```python
from build123d import *

# Parameters (mm, degrees)
F0_W     = 76.2
F0_H     = 50.8
F0_R     = 12.7
F1_DEPTH = 12.7
F2_W     = 6.35
F2_H     = 50.8
F3_DEPTH = 2.54
F5_DEPTH = 50.8
F6_R     = 3.175
F7_DEPTH = 12.7


with BuildPart() as f1:
    # F0 (on Top) → F1 (new body)
    with BuildSketch(Plane.XY):
        Rectangle(F0_W, F0_H)
        Circle(F0_R, mode=Mode.SUBTRACT)
    extrude(amount=F1_DEPTH)

    # F2 (on face) → F3 (cut)
    with BuildSketch(Plane.XY.offset(12.7)):
        with BuildLine():
            ThreePointArc((6.35, 10.9985226281), (0, 12.7), (-6.35, 10.9985226281))
            Line((-6.35, 10.9985226281), (-6.35, -10.9985226281))
            ThreePointArc((-6.35, -10.9985226281), (0, -12.7), (6.35, -10.9985226281))
            Line((6.35, -10.9985226281), (6.35, 10.9985226281))
        make_face()
        with Locations((-32.385, 0)):
            Rectangle(F2_W, F2_H)
        with BuildLine():
            Line((-6.35, -10.9985226281), (-6.35, -25.4))
            Line((-6.35, -25.4), (6.35, -25.4))
            Line((6.35, -25.4), (6.35, -10.9985226281))
            ThreePointArc((6.35, -10.9985226281), (0, -12.7), (-6.35, -10.9985226281))
        make_face()
        with BuildLine():
            Line((6.35, 25.4), (-6.35, 25.4))
            Line((-6.35, 25.4), (-6.35, 10.9985226281))
            ThreePointArc((-6.35, 10.9985226281), (0, 12.7), (6.35, 10.9985226281))
            Line((6.35, 10.9985226281), (6.35, 25.4))
        make_face()
    extrude(amount=-F3_DEPTH, mode=Mode.SUBTRACT)

    # F4 (on face) → F5 (cut, through all)
    with BuildSketch(Plane.XZ.offset(25.4)):
        Polygon((31.75, 12.7), (19.05, 12.7), (16.1170606325, 7.62), (34.6829393675, 7.62), align=None)
    extrude(amount=-F5_DEPTH, mode=Mode.SUBTRACT)

    # F6 (on face) → F7 (join)
    with BuildSketch(Plane.YZ.offset(38.1)):
        with Locations((0, 6.35)):
            Circle(F6_R)
    extrude(amount=F7_DEPTH)


solid = f1.part
```
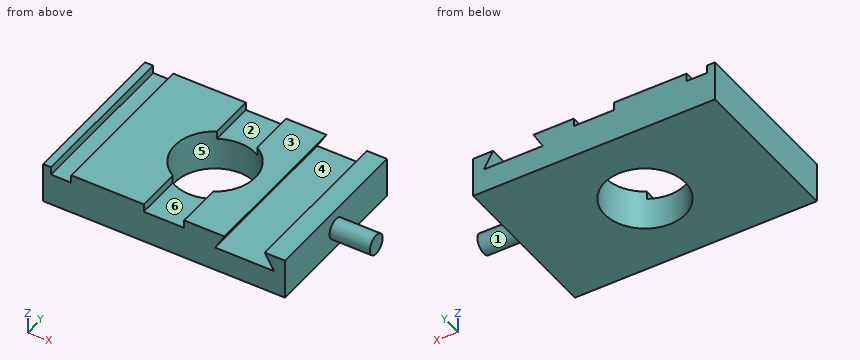
The model under review builds one solid part; all positions refer to its coordinate system, in mm. Face numbers are marked on the shaded views. A direction names the side the tool comes from. Round coordinates to 2 decimals unless told otherwise and drop trailing zeros. Order: outer loops, then holes, each group sorted by start corner. A loop starts at its lowest first (then second) coordinate and runs counter-clockwise, first axis right, second up.
Item 1: Add section A-A, the plane y = 0. State the section outline as (x, z) points (3 decimals).
Working result:
outline: (-38.1, 0) - (-12.7, 0) - (-12.7, 12.7) - (-29.21, 12.7) - (-29.21, 10.16) - (-35.56, 10.16) - (-35.56, 12.7) - (-38.1, 12.7) - close; (12.7, 0) - (38.1, 0) - (38.1, 3.175) - (50.8, 3.175) - (50.8, 9.525) - (38.1, 9.525) - (38.1, 12.7) - (31.75, 12.7) - (34.683, 7.62) - (16.117, 7.62) - (19.05, 12.7) - (12.7, 12.7) - close
Item 2: To check wall thickness, follow probe 1 along Y at (x, z) = (0, 2.5); probe 2 along X at (y, z) = (9, 8.5); probe 3 along X at (y, z) = (0, 3.5). State the ranges of each line that lie inside material, in increasing order.
Working result:
probe 1: y = -25.4 to -12.7, 12.7 to 25.4
probe 2: x = -38.1 to -8.96, 8.96 to 16.63, 34.17 to 38.1
probe 3: x = -38.1 to -12.7, 12.7 to 50.8
Item 3: Draft analysis for pull direction Z (two halves, no side actions). For the marked faces 4, 5 and 6, state which applies: released by +Z, released by -Z, zero draft, split by the parting line, or undercut.
Working result:
face 4: undercut
face 5: zero draft
face 6: released by +Z
Item 4: Add section C-C, the plane x = 0. State the section outline as (y, z) points.
Working result:
outline: (-25.4, 0) - (-12.7, 0) - (-12.7, 10.16) - (-25.4, 10.16) - close; (12.7, 0) - (25.4, 0) - (25.4, 10.16) - (12.7, 10.16) - close
Item 5: For pin 1 (2 mm diameter, centred on y = 20.5, z = 12, fed in from +X); pin 2 (6.5 mm diameter, centred on x = -1.5, y = 16.5, fed in from +Z); pin 3 (9.5 mm diameter, centred on x = 25.5, y = 3.5, fed in from +Z); pin 4 (1 mm diameter, centred on x = -12.5, y = 1.5, fed in from -Z), all flat-tipped, find the tip position at first contact; note any pin that passes through.
Working result:
pin 1: stops at x = 38.1
pin 2: stops at z = 10.16
pin 3: stops at z = 7.62
pin 4: stops at z = 0
Item 6: Add section B-B, the plane z = 6.35. State the section outline as (x, y) points (3 decimals), and give its area (3 significant figures).
Working result:
outline: (-38.1, -25.4) - (38.1, -25.4) - (38.1, -3.175) - (50.8, -3.175) - (50.8, 3.175) - (38.1, 3.175) - (38.1, 25.4) - (-38.1, 25.4) - close; hole circle Ø25.4 at (0, 0)
area: 3,440 mm2
Item 7: Machinability: for the marked faces 1, 2 and 3, which of the approach directions +Z, -Z, +X, -X, +Y, -Y give a long, thin tool a straight path to every point of the face, cutting with its end or side? Answer none if there is none.
Working result:
face 1: +X
face 2: +Z, +Y, -Y
face 3: +Z, +X, -X, +Y, -Y
Item 8: Add section D-D, the plane y = -7.5. State the section outline as (x, z) points.
Working result:
outline: (-38.1, 0) - (-10.25, 0) - (-10.25, 12.7) - (-29.21, 12.7) - (-29.21, 10.16) - (-35.56, 10.16) - (-35.56, 12.7) - (-38.1, 12.7) - close; (10.25, 0) - (38.1, 0) - (38.1, 12.7) - (31.75, 12.7) - (34.68, 7.62) - (16.12, 7.62) - (19.05, 12.7) - (10.25, 12.7) - close
